Work out the finished part from the listing and answer in its coordinate system (mm). Round coordinates to 2 decimals unless told otherwise and drop trailing zeros. Order: outer loops, then holes, each group sorted by start corner. A loop starts at its lowest first (then second) coordinate and runs counter-clockwise, first axis right, second up. Notation, with made-up numbers: (-2.5, 89.5) - (54.5, 89.5) arc R23 cw to (54.5, 106.5) - close; hole circle Ø7 at (3, -22.5). An arc over 180 degrees is marked (long way). Use CSV: the item, a comma, the result in double quotes.
from build123d import *

# Parameters (mm, degrees)
F0_W     = 200
F0_H     = 200
F0_W_2   = 300
F0_H_2   = 150
F1_DEPTH = 200
F2_W     = 10
F2_H     = 180
F3_DEPTH = 100
F4_R     = 34.8685713904
F5_DEPTH = 10


with BuildPart() as f1:
    # F0 (on Front) → F1 (new body)
    with BuildSketch(Plane.XZ):
        Polygon((-37.6349433511, 340.9807319556), (-237.6349433511, 190.9807319556), (-37.6349433511, 190.9807319556), align=None)
        with Locations((-137.6349433511, 90.9807319556)):
            Rectangle(F0_W, F0_H)
        with Locations((112.3650566489, 265.9807319556)):
            Rectangle(F0_W_2, F0_H_2)
        with Locations((112.3650566489, 90.9807319556)):
            Rectangle(F0_W_2, F0_H)
        Polygon((262.3650566489, 340.9807319556), (262.3650566489, 190.9807319556), (462.3650566489, 190.9807319556), align=None)
        with Locations((362.3650566489, 90.9807319556)):
            Rectangle(F0_W, F0_H)
    extrude(amount=F1_DEPTH)

    # F2 (on face) → F3 (cut)
    with BuildSketch(Plane.XZ.offset(200)):
        with Locations((-22.6349433511, 90.9807319556)):
            Rectangle(F2_W, F2_H)
        with Locations((-2.6349433511, 90.9807319556)):
            Rectangle(F2_W, F2_H)
        with Locations((17.3650566489, 90.9807319556)):
            Rectangle(F2_W, F2_H)
        with Locations((37.3650566489, 90.9807319556)):
            Rectangle(F2_W, F2_H)
        with Locations((57.3650566489, 90.9807319556)):
            Rectangle(F2_W, F2_H)
        with Locations((77.3650566489, 90.9807319556)):
            Rectangle(F2_W, F2_H)
        with Locations((97.3650566489, 90.9807319556)):
            Rectangle(F2_W, F2_H)
        with Locations((117.3650566489, 90.9807319556)):
            Rectangle(F2_W, F2_H)
        with Locations((137.3650566489, 90.9807319556)):
            Rectangle(F2_W, F2_H)
        with Locations((157.3650566489, 90.9807319556)):
            Rectangle(F2_W, F2_H)
        with Locations((177.3650566489, 90.9807319556)):
            Rectangle(F2_W, F2_H)
        with Locations((197.3650566489, 90.9807319556)):
            Rectangle(F2_W, F2_H)
        with Locations((217.3650566489, 90.9807319556)):
            Rectangle(F2_W, F2_H)
        with Locations((237.3650566489, 90.9807319556)):
            Rectangle(F2_W, F2_H)
    extrude(amount=-F3_DEPTH, mode=Mode.SUBTRACT)

    # F4 (on face) → F5 (join)
    with BuildSketch(Plane.XZ.offset(200)):
        with Locations((-136.0715925694, 98.517626524)):
            Circle(F4_R)
    extrude(amount=F5_DEPTH)


solid = f1.part
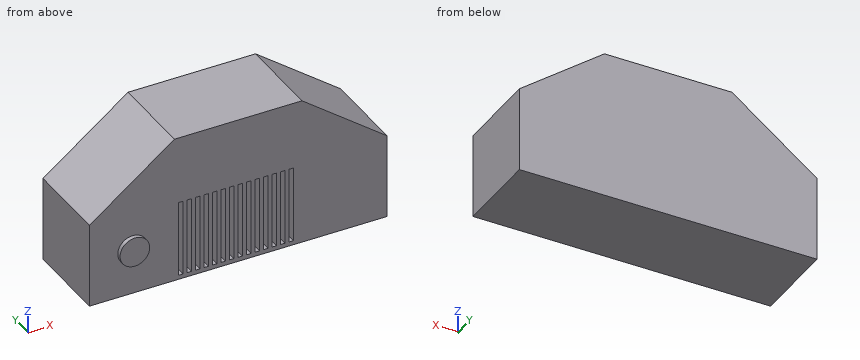
(1) Find section A-A (y = -136). State how many separate pieces and enclosed holes the cut face has, and give its area (3 significant figures).
Findings below:
separate pieces,"1"
enclosed holes,"14"
area,"190,000 mm²"
(2) Find the intervals of material crossed by L1, parallel to Z at x = 78, y = -101; L2, parallel to Y at x = 116, z = 230; L3, parallel to Y at x = 236, z = 115, in increasing order. Write a range as from..to.
Findings below:
L1,"z = -9.02..0.98, 180.98..340.98"
L2,"y = -200..0"
L3,"y = -100..0"
(3) Find section B-B (y = -49.5). Determine the outline of the cut face in (x, z).
Findings below:
outline,"(-237.63, -9.02) - (462.37, -9.02) - (462.37, 190.98) - (262.37, 340.98) - (-37.63, 340.98) - (-237.63, 190.98) - close"
(4) Find section C-C (x = 407). Determine the outline of the cut face in (y, z), and give its area (3 significant figures).
Findings below:
outline,"(-200, -9.02) - (0, -9.02) - (0, 232.5) - (-200, 232.5) - close"
area,"48,300 mm²"
(5) Find section D-D (z = 303). Determine the outline of the cut face in (x, y).
Findings below:
outline,"(-88.28, -200) - (313.01, -200) - (313.01, 0) - (-88.28, 0) - close"
(6) Each of these flat-tipped pins is pushed along its axis until it touches: pin 1 (1.5 mm diameter, centred on x = 26, z = 148, fed in from -Y); pin 2 (8 mm diameter, centred on x = -44.5, y = -163.5, fed in from +Z); pin 3 (5 mm diameter, centred on x = 38, z = 103, fed in from -Y). Where does it stop, or does it pass through?
Findings below:
pin 1,"stops at y = -200"
pin 2,"stops at z = 338.83"
pin 3,"stops at y = -100"
